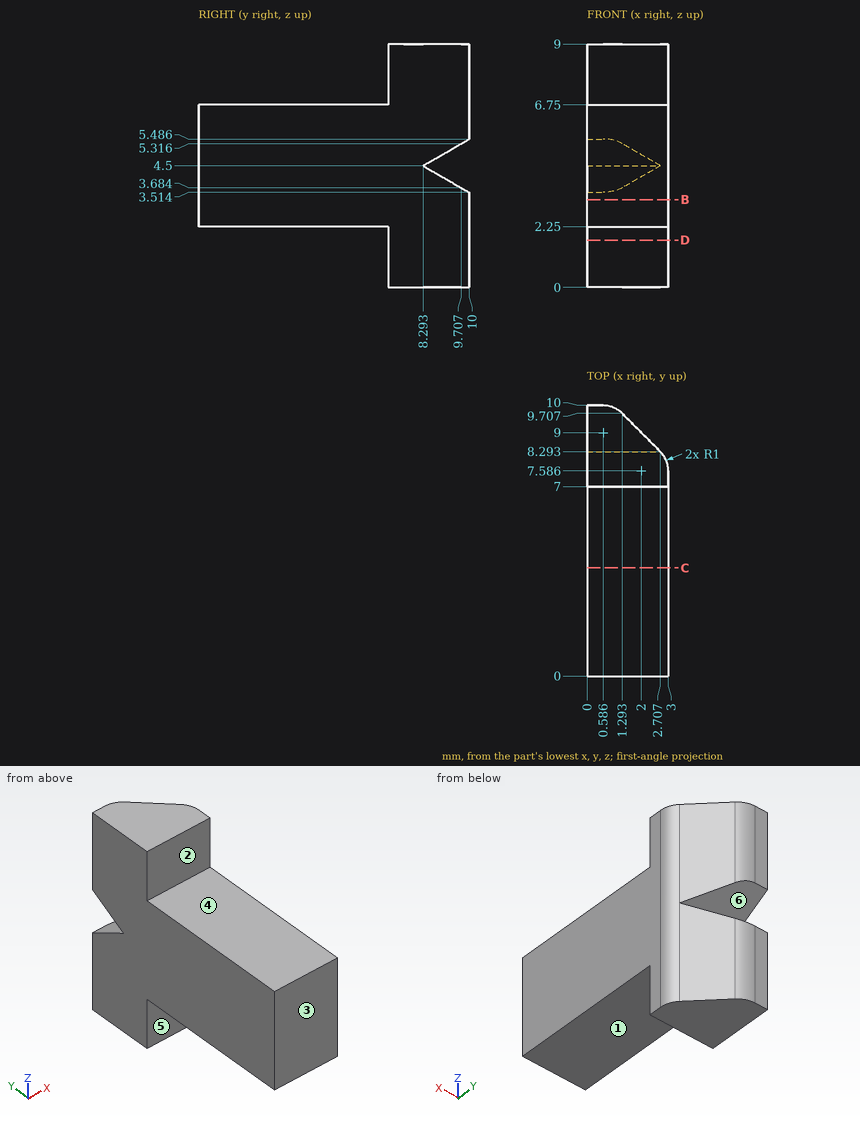
The figure shows three views and two pictorial views of one solid part (mm, origin at its lowest corner). Answer the questions. A direction names the side the tool comes from. Coordinates: 2 decimals unless noted, no trailing zeros. Loops run counter-clockwise (first coordinate to the right, second up) from the corner with the lowest first, then second, coordinate; pieces in that order, holes last. Notation, with made-up numbers: (48, 62.25) -> (62, 62.25) arc R20 cw to (62, 99.25) -> close; hole circle Ø1 at (-22, -27). An arc over 180 degrees is marked (long way). Return JSON: item names as keys, results as strings. Group by question number.
(1) Which of the six approach directions +Z, -Z, +X, -X, +Y, -Y give full straight-line access (tool end or side, diameter ignored) to the marked faces 1, 2 and 3?
(2) A cutting plane is placed at C-C on y = 4. Write down the section's boundary in (x, z).
(3) Find the intervals of material crossed by probe 1 along Z at (x, y) = (1.1, 6.5); probe 2 along Y at (x, z) = (2, 1.5); probe 3 along X at (y, z) = (8.75, 7), in increasing order. Write a range as from..to.
(4) Given pin 1 Ø0.7 at (x, z) = (1, 0.5) entering from -Y; pin 2 Ø1.5 at (x, y) = (1, 4) entering from +Z, each flat-ended and moving along its own axis, determine where each tip first touches the part or whether it passes through.
(5) A cutting plane is placed at D-D on z = 1.75. Write down the section's boundary in (x, y) (1 decimal).
(6) Determine the mould class of the marked faces 4, 5 and 6 for opening direction Z: released by +Z, released by -Z, zero draft, split by the parting line, or undercut.
(7) A cutting plane is placed at B-B on z = 3.25. Write down the section's boundary in (x, y) (1 decimal).
The answers:
{
 "1": {"face 1": "-Z, +X, -X, -Y", "face 2": "+Z, +X, -X, -Y", "face 3": "+Z, -Z, +X, -X, -Y"},
 "2": {"outline": "(0, 2.25) -> (3, 2.25) -> (3, 6.75) -> (0, 6.75) -> close"},
 "3": {"probe 1": "z = 2.25..6.75", "probe 2": "y = 7..9", "probe 3": "x = 0..2.25"},
 "4": {"pin 1": "stops at y = 7", "pin 2": "stops at z = 6.75"},
 "5": {"outline": "(0, 7) -> (3, 7) -> (3, 7.6) arc R1 ccw to (2.7, 8.3) -> (1.3, 9.7) arc R1 ccw to (0.6, 10) -> (0, 10) -> close"},
 "6": {"face 4": "released by +Z", "face 5": "zero draft", "face 6": "undercut"},
 "7": {"outline": "(0, 0) -> (3, 0) -> (3, 7.6) arc R1 ccw to (2.7, 8.3) -> (1.3, 9.7) arc R1 ccw to (0.6, 10) -> (0, 10) -> close"}
}
